from build123d import *

# Parameters (mm, degrees)
F1_DEPTH = 12.7
F0_R     = 9.525
F2_DEPTH = 22.225


with BuildPart() as f1:
    # F0 (on Top) → F1 (new body, symmetric)
    with BuildSketch(Plane.XY):
        with BuildLine():
            ThreePointArc((88.7222, 14.2875), (98.8249881362, 10.1027881362), (103.0097, 0))
            Line((103.0097, 0), (110.9472, 0))
            ThreePointArc((110.9472, 0), (104.4376482119, 15.7154482119), (88.7222, 22.225))
            Line((88.7222, 22.225), (88.7222, 14.2875))
        make_face()
        with BuildLine():
            Line((66.4972, 0), (74.4347, 0))
            ThreePointArc((74.4347, 0), (78.6194118638, 10.1027881362), (88.7222, 14.2875))
            Line((88.7222, 14.2875), (88.7222, 22.225))
            ThreePointArc((88.7222, 22.225), (73.0067517881, 15.7154482119), (66.4972, 0))
        make_face()
        with BuildLine():
            ThreePointArc((88.7222, 22.225), (104.4376482119, 15.7154482119), (110.9472, 0))
            Line((110.9472, 0), (125.222, 0))
            ThreePointArc((125.222, 0), (123.0207927202, 12.4836668274), (116.682668965, 23.461619196))
            ThreePointArc((116.682668965, 23.461619196), (111.4870759361, 37.3222969765), (116.1485113735, 51.3716241887))
            ThreePointArc((116.1485113735, 51.3716241887), (101.3767802444, 45.3853872913), (88.852182223, 55.2430501556))
            ThreePointArc((88.852182223, 55.2430501556), (89.9420456997, 51.5031131444), (90.3097, 47.625))
            ThreePointArc((90.3097, 47.625), (89.9089336946, 43.5776532611), (88.7222, 39.6875))
            Line((88.7222, 39.6875), (88.7222, 22.225))
        make_face()
        with BuildLine():
            Line((125.222, 0), (110.9472, 0))
            ThreePointArc((110.9472, 0), (88.7222, -22.225), (66.4972, 0))
            Line((66.4972, 0), (44.45, 0))
            ThreePointArc((44.45, 0), (38.8703841816, -13.4703841816), (25.4, -19.05))
            Line((25.4, -19.05), (0, -19.05))
            ThreePointArc((0, -19.05), (-1.7112193853, -18.9729868027), (-3.4086029201, -18.7425698914))
            Line((-3.4086029201, -18.7425698914), (82.4730946464, -34.3613781342))
            ThreePointArc((82.4730946464, -34.3613781342), (100.6094978328, -32.8397286109), (115.5177113754, -22.3999150697))
            ThreePointArc((115.5177113754, -22.3999150697), (125.0932774359, -16.9217551289), (135.9264520761, -19.005988544))
            ThreePointArc((135.9264520761, -19.005988544), (128.0821503671, -10.9065679155), (125.222, 0))
        make_face()
        with BuildLine():
            Line((44.45, 0), (66.4972, 0))
            ThreePointArc((66.4972, 0), (73.0067517881, 15.7154482119), (88.7222, 22.225))
            Line((88.7222, 22.225), (88.7222, 39.6875))
            ThreePointArc((88.7222, 39.6875), (63.1687863903, 28.0389841297), (49.6579571791, 52.6585365854))
            ThreePointArc((49.6579571791, 52.6585365854), (33.8807382573, 28.4450035745), (6.5503572572, 19.05))
            Line((6.5503572572, 19.05), (25.4, 19.05))
            ThreePointArc((25.4, 19.05), (38.8703841816, 13.4703841816), (44.45, 0))
        make_face()
    extrude(amount=F1_DEPTH, both=True)

    # F0 (on Top) → F2 (join, symmetric)
    with BuildSketch(Plane.XY):
        with BuildLine():
            ThreePointArc((88.7222, 14.2875), (98.8249881362, 10.1027881362), (103.0097, 0))
            Line((103.0097, 0), (110.9472, 0))
            ThreePointArc((110.9472, 0), (104.4376482119, 15.7154482119), (88.7222, 22.225))
            Line((88.7222, 22.225), (88.7222, 14.2875))
        make_face()
        with BuildLine():
            Line((110.9472, 0), (103.0097, 0))
            ThreePointArc((103.0097, 0), (88.7222, -14.2875), (74.4347, 0))
            Line((74.4347, 0), (66.4972, 0))
            ThreePointArc((66.4972, 0), (88.7222, -22.225), (110.9472, 0))
        make_face()
        with BuildLine():
            Line((66.4972, 0), (74.4347, 0))
            ThreePointArc((74.4347, 0), (78.6194118638, 10.1027881362), (88.7222, 14.2875))
            Line((88.7222, 14.2875), (88.7222, 22.225))
            ThreePointArc((88.7222, 22.225), (73.0067517881, 15.7154482119), (66.4972, 0))
        make_face()
        with BuildLine():
            ThreePointArc((116.682668965, 23.461619196), (123.0207927202, 12.4836668274), (125.222, 0))
            Line((125.222, 0), (136.3218, 0))
            ThreePointArc((136.3218, 0), (133.4511928724, 16.2800220142), (125.1856090747, 30.596433106))
            ThreePointArc((125.1856090747, 30.596433106), (126.556865998, 46.2699714599), (142.2304043519, 44.8987145366))
            ThreePointArc((142.2304043519, 44.8987145366), (154.3597295619, 23.8901070113), (158.5722, 0))
            Line((158.5722, 0), (169.672, 0))
            ThreePointArc((169.672, 0), (164.7901297141, 27.6864621982), (150.7333444616, 52.0335284466))
            ThreePointArc((150.7333444616, 52.0335284466), (133.2827298684, 59.9685045985), (116.1485113735, 51.3716241887))
            ThreePointArc((116.1485113735, 51.3716241887), (111.4870759361, 37.3222969765), (116.682668965, 23.461619196))
        make_face()
        with BuildLine():
            Line((136.3218, 0), (125.222, 0))
            ThreePointArc((125.222, 0), (128.0821503671, -10.9065679155), (135.9264520761, -19.005988544))
            ThreePointArc((135.9264520761, -19.005988544), (158.3535679155, -19.3648496329), (169.672, 0))
            Line((169.672, 0), (158.5722, 0))
            ThreePointArc((158.5722, 0), (147.447, -11.1252), (136.3218, 0))
        make_face()
        with BuildLine():
            ThreePointArc((25.4, -19.05), (38.8703841816, -13.4703841816), (44.45, 0))
            ThreePointArc((44.45, 0), (38.8703841816, 13.4703841816), (25.4, 19.05))
            Line((25.4, 19.05), (6.5503572572, 19.05))
            Line((6.5503572572, 19.05), (0, 19.05))
            ThreePointArc((0, 19.05), (-18.9729868027, 1.7112193853), (-3.4086029201, -18.7425698914))
            ThreePointArc((-3.4086029201, -18.7425698914), (-1.7112193853, -18.9729868027), (0, -19.05))
            Line((0, -19.05), (25.4, -19.05))
        make_face()
        with BuildLine():
            ThreePointArc((25.4, 11.0998), (33.2487438498, 7.8487438498), (36.4998, 0))
            ThreePointArc((36.4998, 0), (33.2487438498, -7.8487438498), (25.4, -11.0998))
            Line((25.4, -11.0998), (0, -11.0998))
            ThreePointArc((0, -11.0998), (-11.0998, 0), (0, 11.0998))
            Line((0, 11.0998), (25.4, 11.0998))
        make_face(mode=Mode.SUBTRACT)
        with BuildLine():
            ThreePointArc((49.6579571791, 52.6585365854), (63.1687863903, 28.0389841297), (88.7222, 39.6875))
            ThreePointArc((88.7222, 39.6875), (89.9089336946, 43.5776532611), (90.3097, 47.625))
            ThreePointArc((90.3097, 47.625), (89.9420456997, 51.5031131444), (88.852182223, 55.2430501556))
            ThreePointArc((88.852182223, 55.2430501556), (68.314287895, 68.217777398), (49.6579571791, 52.6585365854))
        make_face()
        with Locations((69.6722, 47.625)):
            Circle(F0_R, mode=Mode.SUBTRACT)
    extrude(amount=F2_DEPTH, both=True)


solid = f1.part
Verification items for the finished model (mm, model axes). A direction names the side the tool comes from. Give positions to 0.01 mm unless a question says otherwise; leave off trailing zeros. Loops run counter-clockwise (first coordinate to the right, second up) from the corner with the lowest first, then second, coordinate; pieces in that order, holes last.
1) Thickness scan on line 1 along X through (y, z) = (44.5, -12.5); line 2 along Y through (x, z) = (76, -10); line 3 along X through (y, z) = (2.5, -11). Record the ranges inside material, lowest first.
2) Depth check by flat-ended pin: pin 1 Ø10.5 at (x, z) = (6.5, -16.5) entering from -Y; pin 2 Ø5 at (x, z) = (50, 13.5) entering from +Y; pin 3 Ø7.5 at (x, z) = (8, 3) entering from -Y. Enter the tip coordinate at first touch or a pass-through.
3) Set-up check for faces 4 (the cylindrical face through (122.96, 12.65, -17.53)), 5 (the flat face through (13, -19.05, 17)), 6 (the cylindrical face through (122.96, 12.65, 17.4)), 7 (the flat face through (13, -19.05, -18)): record each of +Z, -Z, +X, -X, +Y, -Y from which the full face is reachable in a straight line by a thin tool's end or side.
4) Sectioned sample at A-A, the plane z = 16. Count the separate pieces of the cut face and the enclosed holes in it, then the cut area to 3 significant figures.
5) Sectioned sample at B-B, the plane y = 41.5. Enter the section's corners in (x, z) (3 decimals).
6) Sectioned sample at C-C, the plane x = -7. Enter the section's corners in (y, z) (3 decimals), then the cut area to 3 significant figures.
7) Draft check along Y on faces 1 (the cylindrical face through (-19.045, 0.419, 0.311)), 2 (the flat face through (13, 11.1, 0)), 3 (the cylindrical face through (124.94, -16.95, 0.18)). Enter one of: pulls with the +Y half, pulls with the -Y half, needs draft (parallel to the pull), parting line crosses it, or undercut.
Answers:
1. line 1: x = 46.73 to 60.67, 78.67 to 124.87, 142.56 to 156.34
1. line 2: y = -33.18 to -6.5, 6.5 to 40.51, 54.74 to 67.27
1. line 3: x = -18.89 to -10.81, 36.21 to 74.66, 102.79 to 136.26, 158.53 to 169.63
2. pin 1: stops at y = -21.2
2. pin 2: stops at y = 59.07
2. pin 3: stops at y = -21.5
3. face 4: -Z, -Y
3. face 5: +Z, -X, -Y
3. face 6: +Z, -Y
3. face 7: -Z, -X, -Y
4. separate pieces: 4
4. enclosed holes: 4
4. area: 5,190 mm2
5. outline: (45.174, -12.7) - (49.965, -12.7) - (49.965, -22.225) - (62.378, -22.225) - (62.378, 22.225) - (49.965, 22.225) - (49.965, 12.7) - (45.174, 12.7) - close; (76.967, -22.225) - (89.38, -22.225) - (89.38, -12.7) - (111.802, -12.7) - (111.802, -22.225) - (123.235, -22.225) - (123.235, 22.225) - (111.802, 22.225) - (111.802, 12.7) - (89.38, 12.7) - (89.38, 22.225) - (76.967, 22.225) - close; (144.907, -22.225) - (158.225, -22.225) - (158.225, 22.225) - (144.907, 22.225) - close
6. outline: (-17.717, -22.225) - (-8.614, -22.225) - (-8.614, 22.225) - (-17.717, 22.225) - close; (8.614, -22.225) - (17.717, -22.225) - (17.717, 22.225) - (8.614, 22.225) - close
6. area: 809 mm2
7. face 1: parting line crosses it
7. face 2: undercut
7. face 3: pulls with the -Y half
